Check sheet for the drawn part. Datum: minimum x, y, z corner. Units: mm. A direction names the side the tool comes from. Give positions to 0.01 mm unless a question says otherwise; leave off trailing zeros. Write each loop counter-clockwise with the first axis right and the second up, starting at its lowest first coordinate (ties: lowest second). Pieces come first, ordered by that corner, then holes. Notation, with made-up numbers: M -26.75,74 L 14.25,74 A23 cw 14.25,91 Z; hole C -36,37 d6. An arc over 180 degrees is marked long. Write item = value, one per line. Start each with the question number.
1) Sectioned sample at A-A, the plane y = 18.5. Record the cut outline in (x, z), then the cut area to 3 significant figures.
2) Set-up check for the marked faces 1 and 2: record each of +Z, -Z, +X, -X, +Y, -Y from which the full face is reachable in a straight line by a thin tool's end or side.
3) Gauge pin test, flat ends, axial feed: pin 1 (2 mm diameter, centred on x = 6, y = 33.5, fed in from +Z); pin 2 (4 mm diameter, centred on x = 2.5, y = 23.5, fed in from +Z); pin 3 (1.5 mm diameter, centred on x = 4.5, z = 6, fed in from -Y). Record the tip position at first contact, or that the pin passes through.
4) Scan lines: L1, parallel to Z at x = 3.75, y = 4.5; L2, parallel to Z at x = 3.75, y = 36. Record each from-to range of solid material in increasing order.
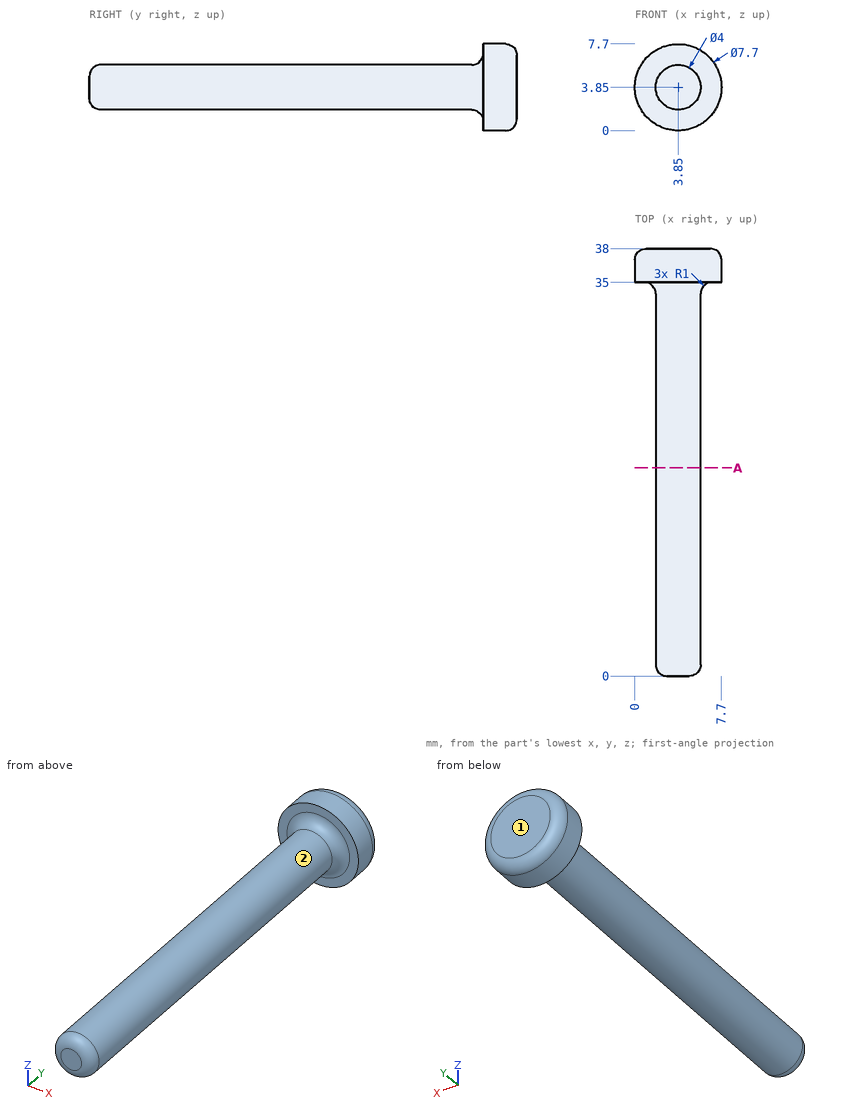
Data:
q1.outline = C 3.85,3.85 d4
q1.area = 12.6 mm2
q2.face_1 = +Z, -Z, +X, -X, +Y
q2.face_2 = -Y
q3.pin_1 = 5.49
q3.pin_2 = 5.85
q3.pin_3 = 0.13
q4.L1 = 1.85 to 5.85
q4.L2 = 0 to 7.7
